Build history of the part. All positions in model axes, mm. Face numbers are marked on the shaded views. A direction names the side the tool comes from. Round coordinates to 2 decimals unless told otherwise and drop trailing zeros. Write each loop counter-clockwise with the first axis right and the second up, starting at its lowest first coordinate (ties: lowest second). Pieces come first, ordered by that corner, then holes. Notation, with made-up numbers: M 31,-28 L 66,-28 A26 ccw 66,6 Z; hole C 49,10 d1. An arc over 180 degrees is marked long. Write item = value, one per line. Start each with the question number.
Q1. Pull direction X, two halves, no side cores. Call the marked faces 6, 7 and 8: released by +X, released by -X, zero draft, split by the parting line, or undercut.
Q2. Band-saw the part on D-D on y = 12. Write the cut outline in (x, z).
Q3. Band-saw the part on C-C on z = 7. Write the cut outline in (x, y).
Q4. Probe L1, parallel to X at y = 24.3, z = 3 (3 decimals); L2, parallel to Y at x = 7.25, z = 4.3; L3, parallel to X at y = 2.5, z = 2.5. List the from-to ranges inside material, lowest first.
Q5. Drop flat-ended pins along their axis: P1, Ø1, axis at x = 3.5, z = 3, coming from the +Y side; P2, Ø6, axis at x = 7.25, y = 7, coming from the -Z side; P3, Ø2.5, axis at x = 3.3, z = 3, coming from the -Y side; P4, Ø1.5, axis at x = 17, z = 3.5, coming from the +Y side. Give the stop position or say it passes through.
Q6. Band-saw the part on A-A on y = 19. Write the cut outline in (x, z).
Q7. Band-saw the part on B-B on x = 7.25. Write the cut outline in (y, z).
Q8. Tool access for the marked faces 1, 2, 3, 4 and 5: list every direction of +Z, -Z, +X, -X, +Y, -Y with a clear straight run to the whole face (end or side of a thin tool).
```python
from build123d import *

# Parameters (mm, degrees)
SKETCH1_W                      = 15.6
SKETCH1_H                      = 26
BOSS_EXTRUDE1_DEPTH            = 6
SKETCH2_R                      = 1.675
CUT_EXTRUDE1_DEPTH             = 4.5
CUT_EXTRUDE2_START             = -4.5
SKETCH3_R                      = 1.675
CUT_EXTRUDE2_DEPTH             = 4.5
SKETCH4_W                      = 36.5
SKETCH4_H                      = 20
BOSS_EXTRUDE2_DEPTH            = 3
CBORE_FOR_M3_SHCS4_D           = 3.2
CBORE_FOR_M3_SHCS4_CBORE_D     = 6.6
CBORE_FOR_M3_SHCS4_CBORE_DEPTH = 3


with BuildPart() as part:
    # Sketch1 → Boss-Extrude1 (new body)
    with BuildSketch(Plane.XY):
        with Locations((7.8, 13)):
            Rectangle(SKETCH1_W, SKETCH1_H)
    extrude(amount=BOSS_EXTRUDE1_DEPTH)

    # Sketch2 → Cut-Extrude1 (cut)
    with BuildSketch(Plane(origin=(0, 26, 0), x_dir=(1, 0, 0), z_dir=(0, 1, 0))):
        with Locations(Location((3.3, -3, 0), (0, 0, 270))):
            Circle(SKETCH2_R)
        with Locations(Location((12.3, -3, 0), (0, 0, 270))):
            Circle(SKETCH2_R)
    extrude(amount=-CUT_EXTRUDE1_DEPTH, mode=Mode.SUBTRACT)

    # Sketch3 → Cut-Extrude2 (cut)
    with BuildSketch(Plane.XZ.offset(CUT_EXTRUDE2_START)):
        with Locations(Location((12.3, 3, 0), (0, 0, 90))):
            Circle(SKETCH3_R)
        with Locations(Location((3.3, 3, 0), (0, 0, 90))):
            Circle(SKETCH3_R)
    extrude(amount=CUT_EXTRUDE2_DEPTH, mode=Mode.SUBTRACT)

    # Sketch4 → Boss-Extrude2 (add)
    with BuildSketch(Plane.XY.offset(6)):
        with Locations((18.25, 13)):
            Rectangle(SKETCH4_W, SKETCH4_H)
    extrude(amount=BOSS_EXTRUDE2_DEPTH)

    # CBORE for M3 SHCS4 (through all)
    with Locations(Plane(origin=(0, 0, 0), x_dir=(-1, 0, 0), z_dir=(0, 0, -1))):
        with Locations((-33.25, 19), (-7.25, 19), (-7.25, 7), (-33.25, 7)):
            CounterBoreHole(CBORE_FOR_M3_SHCS4_D / 2, CBORE_FOR_M3_SHCS4_CBORE_D / 2, CBORE_FOR_M3_SHCS4_CBORE_DEPTH)


solid = part.part
```
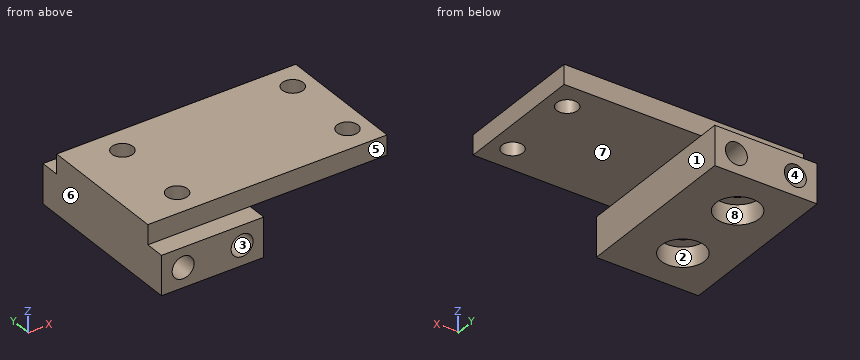
Conclusion:
q1.face_6 = released by -X
q1.face_7 = zero draft
q1.face_8 = undercut
q2.outline = M 0,0 L 15.6,0 L 15.6,6 L 36.5,6 L 36.5,9 L 0,9 Z
q3.outline = M 0,3 L 36.5,3 L 36.5,23 L 0,23 Z; hole C 7.25,7 d3.2; hole C 7.25,19 d3.2; hole C 33.25,7 d3.2; hole C 33.25,19 d3.2
q4.L1 = 0 to 1.625, 4.975 to 10.625, 13.975 to 15.6
q4.L2 = 0 to 5.4, 8.6 to 17.4, 20.6 to 26
q4.L3 = 0 to 1.7, 4.9 to 10.7, 13.9 to 15.6
q5.P1 = 21.5
q5.P2 = 3
q5.P3 = 4.5
q5.P4 = through
q6.outline = M 0,0 L 3.95,0 L 3.95,3 L 5.65,3 L 5.65,9 L 0,9 Z; M 8.85,3 L 10.55,3 L 10.55,0 L 15.6,0 L 15.6,6 L 31.65,6 L 31.65,9 L 8.85,9 Z; M 34.85,6 L 36.5,6 L 36.5,9 L 34.85,9 Z
q7.outline = M 0,0 L 3.7,0 L 3.7,3 L 5.4,3 L 5.4,9 L 3,9 L 3,6 L 0,6 Z; M 8.6,3 L 10.3,3 L 10.3,0 L 15.7,0 L 15.7,3 L 17.4,3 L 17.4,9 L 8.6,9 Z; M 20.6,3 L 22.3,3 L 22.3,0 L 26,0 L 26,6 L 23,6 L 23,9 L 20.6,9 Z
q8.face_1 = -Z, +X, +Y, -Y
q8.face_2 = -Z
q8.face_3 = -Y
q8.face_4 = +Y
q8.face_5 = +Z, +X, -X, -Y
